Input: part model. Units: mm. Frame: model coordinates. A direction names the side the tool comes from. Give positions to 0.01 mm unless a question says otherwise; leave off trailing zeros. Loops run counter-clockwise (first coordinate to the right, second up) from the corner with the lowest first, then second, coordinate; pieces in that order, holes last.
from build123d import *

# Parameters (mm, degrees)
F0_R        = 3.5
F0_R_2      = 46.5
F0_W        = 8
F0_H        = 37
F0_R_3      = 5
F1_DEPTH    = 2
F0_R_4      = 1.5
F2_DEPTH    = 22
F0_W_2      = 38.8732933998
F0_H_2      = 3.6201002002
F0_W_3      = 3
F0_H_3      = 27
F3_DEPTH    = 45
F4_R        = 29.99999
F5_R        = 10
F6_W        = 50
F6_H        = 15
F7_DEPTH    = 5
F8_R        = 5
F0_R_5      = 1
F9_DEPTH    = 8
F10_R       = 1.5
F11_DEPTH   = 25
F12_SIZE2   = 19.99999
F12_SIZE    = 14.99999
F12_2_SIZE2 = 19.99999
F12_2_SIZE  = 14.99999


# Not quite as in the source:
# - a fillet or chamfer is up to 0.001 mm smaller than in the source, because OpenCascade refuses the exact size


with BuildPart() as f1:
    # F0 (on Top) → F1 (new body)
    with BuildSketch(Plane.XY):
        Polygon((126.1267066002, 107), (3, 107), (3, 3), (107, 3), (107, 30), (107, 33), (177, 33), (177, 95), (177, 107), (165, 107), (165, 103.3798997998), (126.1267066002, 103.3798997998), align=None)
        with Locations((17.5, 16.5)):
            Circle(F0_R, mode=Mode.SUBTRACT)
        with Locations((94.5, 16.5)):
            Circle(F0_R, mode=Mode.SUBTRACT)
        with Locations((56, 55)):
            Circle(F0_R_2, mode=Mode.SUBTRACT)
        with Locations((17.5, 93.5)):
            Circle(F0_R, mode=Mode.SUBTRACT)
        with Locations((118, 65)):
            Rectangle(F0_W, F0_H, mode=Mode.SUBTRACT)
        with Locations((171, 65)):
            Rectangle(F0_W, F0_H, mode=Mode.SUBTRACT)
        with Locations((94.5, 93.5)):
            Circle(F0_R, mode=Mode.SUBTRACT)
        with Locations((107, 97)):
            Circle(F0_R_3, mode=Mode.SUBTRACT)
    extrude(amount=F1_DEPTH)

    # F0 (on Top) → F2 (join)
    with BuildSketch(Plane.XY):
        with Locations((118, 65)):
            Rectangle(F0_W, F0_H)
        with Locations((118, 65.5)):
            Circle(F0_R_4, mode=Mode.SUBTRACT)
        with Locations((118, 80.5)):
            Circle(F0_R_4, mode=Mode.SUBTRACT)
        with Locations((171, 65)):
            Rectangle(F0_W, F0_H)
        with Locations((171, 65.5)):
            Circle(F0_R_4, mode=Mode.SUBTRACT)
        with Locations((171, 80.5)):
            Circle(F0_R_4, mode=Mode.SUBTRACT)
    extrude(amount=F2_DEPTH)

    # F0 (on Top) → F3 (join)
    with BuildSketch(Plane.XY):
        Polygon((3, 110), (0, 110), (0, 3), (3, 3), (3, 107), align=None)
        Polygon((165, 110), (3, 110), (3, 107), (126.1267066002, 107), (165, 107), align=None)
        Polygon((3, 3), (0, 3), (0, 0), (110, 0), (110, 3), (107, 3), align=None)
        with Locations((145.5633533001, 105.1899498999)):
            Rectangle(F0_W_2, F0_H_2)
        with Locations((108.5, 16.5)):
            Rectangle(F0_W_3, F0_H_3)
        Polygon((107, 33), (107, 30), (110, 30), (177, 30), (177, 33), align=None)
        Polygon((180, 30), (180, 95), (177, 95), (177, 33), (177, 30), align=None)
    extrude(amount=F3_DEPTH)

    # F4 (radius 30 in the source; OpenCascade refuses exactly that, so slightly less here)
    f4_edges = [f1.edges().sort_by_distance(p)[0] for p in [
        (3, 107, 23.5),
        (3, 3, 23.5),
        (107, 3, 23.5),
    ]]
    fillet(f4_edges, radius=F4_R)

    # F5
    f5_edges = [f1.edges().sort_by_distance(p)[0] for p in [
        (177, 33, 23.5),
        (180, 30, 22.5),
        (110, 30, 22.5),
        (107, 33, 23.5),
        (177, 107, 1),
    ]]
    fillet(f5_edges, radius=F5_R)

    # F6 (on face) → F7 (cut)
    with BuildSketch(Plane.XZ.offset(-30)):
        with Locations((145, 12.5)):
            Rectangle(F6_W, F6_H)
    extrude(amount=-F7_DEPTH, mode=Mode.SUBTRACT)

    # F8
    f8_edges = [f1.edges().sort_by_distance(p)[0] for p in [
        (110, 0, 22.5),
        (0, 0, 22.5),
        (0, 110, 22.5),
    ]]
    fillet(f8_edges, radius=F8_R)

    # F0 (on Top) → F9 (join)
    with BuildSketch(Plane.XY):
        with Locations((94.5, 93.5)):
            Circle(F0_R)
        with Locations((94.5, 93.5)):
            Circle(F0_R_5, mode=Mode.SUBTRACT)
        with Locations((17.5, 93.5)):
            Circle(F0_R)
        with Locations((17.5, 93.5)):
            Circle(F0_R_5, mode=Mode.SUBTRACT)
        with Locations((17.5, 16.5)):
            Circle(F0_R)
        with Locations((17.5, 16.5)):
            Circle(F0_R_5, mode=Mode.SUBTRACT)
        with Locations((94.5, 16.5)):
            Circle(F0_R)
        with Locations((94.5, 16.5)):
            Circle(F0_R_5, mode=Mode.SUBTRACT)
    extrude(amount=F9_DEPTH)

    # F10 (on face) → F11 (cut)
    with BuildSketch(Plane.XY.offset(45)):
        with Locations((6, 104)):
            Circle(F10_R)
        with Locations((6, 6)):
            Circle(F10_R)
        with Locations((104, 6)):
            Circle(F10_R)
    extrude(amount=-F11_DEPTH, mode=Mode.SUBTRACT)

    # F12 (size 15 and 20 in the source; OpenCascade refuses exactly that, so slightly less here)
    f12_edges = [f1.edges().sort_by_distance(p)[0] for p in [
        (118, 46.5, 22),
    ]]
    f12_side = f1.faces().sort_by_distance((118, 83.12145, 22))[0]
    chamfer(f12_edges, length=F12_SIZE, length2=F12_SIZE2, reference=f12_side)

    # F12#2 (size 15 and 20 in the source; OpenCascade refuses exactly that, so slightly less here)
    f12_2_edges = [f1.edges().sort_by_distance(p)[0] for p in [
        (171, 46.5, 22),
    ]]
    f12_2_side = f1.faces().sort_by_distance((171, 83.12145, 22))[0]
    chamfer(f12_2_edges, length=F12_2_SIZE, length2=F12_2_SIZE2, reference=f12_2_side)


solid = f1.part
(1) Mould query, pull axis Y, two halves, no side actions, for faces 4 (the flat face through (54, 0, 22)), 5 (the flat face through (109, 56, 0)), 6 (the flat face through (118, 54, 12)). Classes: +Y half, -Y half, draft (parallel to the pull), parting line (faces both ways), or undercut.
Values follow:
face 4: -Y half
face 5: draft
face 6: undercut
(2) Cut plane A-A (x = 135). Return the cut outline in (y, z).
Values follow:
outline: (30, 0) - (110, 0) - (110, 45) - (103.38, 45) - (103.38, 2) - (33, 2) - (33, 5) - (30, 5) - close; (30, 20) - (33, 20) - (33, 45) - (30, 45) - close
(3) Ray query, probe 1 along X at (y, z) = (76, 18); probe 2 along Y at (x, z) = (52.5, 39.5); probe 3 along X at (y, z) = (55, 20). Return the intervals inside material, ascending.
Values follow:
probe 1: x = 0 to 3, 114 to 122, 167 to 175, 177 to 180
probe 2: y = 0 to 3, 107 to 110
probe 3: x = 0 to 3, 177 to 180
(4) Pin query (flat end, axial travel): pin 1 Ø4 at (x, z) = (171, 11) entering from +Y; pin 2 Ø5 at (x, y) = (118, 80.5) entering from -Z; pin 3 Ø3.5 at (x, z) = (178, 17) entering from +Y; pin 4 Ø2 at (x, y) = (103, 80) entering from +Z. Return the tip coordinate at first contact, or that it passes through.
Values follow:
pin 1: stops at y = 83.5
pin 2: stops at z = 0
pin 3: stops at y = 95
pin 4: stops at z = 2
(5) Cut plane B-B (y = 35.5). Return the cut outline in (x, z), and give its area (3 significant figures).
Values follow:
outline: (0, 0) - (13.79, 0) - (13.79, 2) - (3, 2) - (3, 45) - (0, 45) - close; (98.21, 0) - (178.93, 0) - (178.93, 45) - (173.61, 45) - (173.61, 2) - (98.21, 2) - close
area: 547 mm2
(6) Reachability of faces 1 (the flat face through (145, 30, 2)), 2 (the cylindrical face through (173.99, 35.85, 23.8)), 3 (the flat face through (167, 69, 12)) from +Z, -Z, +X, -X, +Y, -Y: full face, straight path, thin tool, end or side. Return the list, or none.
Values follow:
face 1: +Z, -Z, +X, -Y
face 2: +Z
face 3: +Z, +Y
(7) Cut plane C-C (y = 48.5). Return the cut outline in (x, z), and give its area (3 significant figures).
Values follow:
outline: (0, 0) - (9.96, 0) - (9.96, 2) - (3, 2) - (3, 45) - (0, 45) - close; (102.04, 0) - (180, 0) - (180, 45) - (177, 45) - (177, 2) - (175, 2) - (175, 4.67) - (167, 4.67) - (167, 2) - (122, 2) - (122, 4.67) - (114, 4.67) - (114, 2) - (102.04, 2) - close
area: 476 mm2
